from build123d import *

# Parameters (mm, degrees)
F0_W     = 355.6
F0_H     = 177.8
F1_DEPTH = 19.05
F2_W     = 304.8
F2_H     = 127
F3_DEPTH = 19.05
F5_DEPTH = 19.05


with BuildPart() as f1:
    # F0 (on Top) → F1 (new body)
    with BuildSketch(Plane.XY):
        Rectangle(F0_W, F0_H)
    extrude(amount=F1_DEPTH)

    # F2 (on face) → F3 (join)
    with BuildSketch(Plane.XY.offset(19.05)):
        Rectangle(F2_W, F2_H)
    extrude(amount=F3_DEPTH)

    # F4 (on face) → F5 (cut)
    with BuildSketch(Plane.XY.offset(38.1)):
        with BuildLine():
            ThreePointArc((-137.163756, -34.489753), (-131.58414, -47.960137), (-118.113756, -53.539753))
            Line((-118.113756, -53.539753), (118.113756, -53.539753))
            ThreePointArc((118.113756, -53.539753), (131.58414, -47.960137), (137.163756, -34.489753))
            Line((137.163756, -34.489753), (137.163756, 34.489753))
            ThreePointArc((137.163756, 34.489753), (131.58414, 47.960137), (118.113756, 53.539753))
            Line((118.113756, 53.539753), (-118.113756, 53.539753))
            ThreePointArc((-118.113756, 53.539753), (-131.58414, 47.960137), (-137.163756, 34.489753))
            Line((-137.163756, 34.489753), (-137.163756, -34.489753))
        make_face()
    extrude(amount=-F5_DEPTH, mode=Mode.SUBTRACT)


solid = f1.part
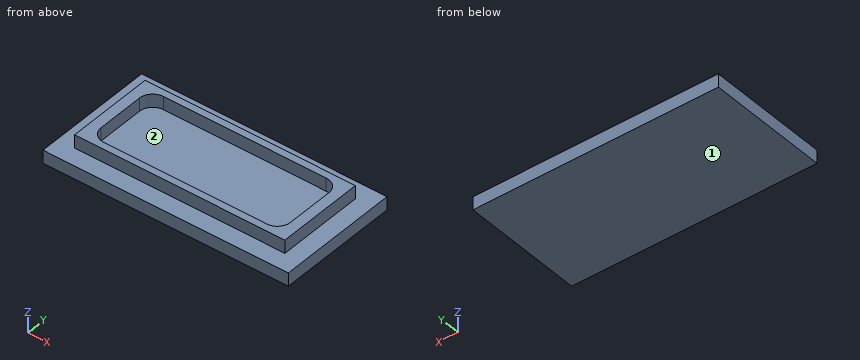
Read the model definition and answer for the solid it produces. Units are mm, in the model's axes. Face numbers are marked on the shaded views. A direction names the side the tool comes from. Round coordinates to 2 decimals unless told otherwise and drop trailing zeros. Write each loop counter-clockwise with the first axis right and the second up, starting at its lowest first coordinate (ties: lowest second). Pieces come first, ordered by that corner, then holes. Notation, with made-up numbers: M 25.5,56 L 70.5,56 A31 ccw 70.5,80 Z; hole C -31,-24 d2. An arc over 180 degrees is marked long. Use a Markdown table: item, result.
1) The part is cut by section C-C (x = -95.5). Write down the section's boundary in (y, z).
Answers follow:
| item | result |
|---|---|
| outline | M -88.9,0 L 88.9,0 L 88.9,19.05 L 63.5,19.05 L 63.5,38.1 L 53.54,38.1 L 53.54,19.05 L -53.54,19.05 L -53.54,38.1 L -63.5,38.1 L -63.5,19.05 L -88.9,19.05 Z |
2) The part is cut by section B-B (y = -58.5). Write down the section's boundary in (x, z), plus the area to 3 significant figures.
Answers follow:
| item | result |
|---|---|
| outline | M -177.8,0 L 177.8,0 L 177.8,19.05 L 152.4,19.05 L 152.4,38.1 L -152.4,38.1 L -152.4,19.05 L -177.8,19.05 Z |
| area | 12,600 mm2 |
3) The part is cut by section A-A (z = 24). Write down the section's boundary in (x, y).
Answers follow:
| item | result |
|---|---|
| outline | M -152.4,-63.5 L 152.4,-63.5 L 152.4,63.5 L -152.4,63.5 Z; hole M -137.16,-34.49 A19.05 ccw -118.11,-53.54 L 118.11,-53.54 A19.05 ccw 137.16,-34.49 L 137.16,34.49 A19.05 ccw 118.11,53.54 L -118.11,53.54 A19.05 ccw -137.16,34.49 Z |
4) The part is cut by section D-D (y = -17). Write down the section's boundary in (x, z).
Answers follow:
| item | result |
|---|---|
| outline | M -177.8,0 L 177.8,0 L 177.8,19.05 L 152.4,19.05 L 152.4,38.1 L 137.16,38.1 L 137.16,19.05 L -137.16,19.05 L -137.16,38.1 L -152.4,38.1 L -152.4,19.05 L -177.8,19.05 Z |
5) A tool of negligible diameter and unlimited length cuts with its end or side. For the marked faces 1 and 2, from which of +Z, -Z, +X, -X, +Y, -Y can it reach the whole face along a straight path? Write none if from no direction.
Answers follow:
| item | result |
|---|---|
| face 1 | -Z, +X, -X, +Y, -Y |
| face 2 | +Z |
6) Straight lines are drawn through the part: line 1 along X through (y, z) = (15.5, 31); line 2 along Z through (x, y) = (-160, 70); line 3 along Y through (x, z) = (23, 33). For each, find the intervals that lie inside material, in ascending order. Write a range as [from, to].
Answers follow:
| item | result |
|---|---|
| line 1 | x = [-152.4, -137.16], [137.16, 152.4] |
| line 2 | z = [0, 19.05] |
| line 3 | y = [-63.5, -53.54], [53.54, 63.5] |
7) Flat-ended cylindrical pins translate along their axes: pin 1 (9.5 mm diameter, centred on x = 43, z = 33, fed in from +Y); pin 2 (2 mm diameter, centred on x = -132, y = -46.5, fed in from -Z); pin 3 (5.5 mm diameter, centred on y = -2, z = 29.5, fed in from -X); pin 4 (8 mm diameter, centred on x = 96.5, y = 24, fed in from +Z). Find the tip coordinate at first contact, or state that the pin passes through.
Answers follow:
| item | result |
|---|---|
| pin 1 | stops at y = 63.5 |
| pin 2 | stops at z = 0 |
| pin 3 | stops at x = -152.4 |
| pin 4 | stops at z = 19.05 |
